Part print with two shaded views. Sizes in mm from the minimum x, y, z corner. A direction names the side the tool comes from. Give positions to 0.01 mm unless a question says otherwise; leave off trailing zeros. Loops run counter-clockwise (first coordinate to the right, second up) from the corner with the lowest first, then second, coordinate; pieces in that order, holes last. Notation, with made-up numbers: M 39,27.25 L 64,27.25 A27 ccw 64,54.25 Z; hole C -7,56 d9. An arc over 180 degrees is marked long. Answer as a JSON object with one key per item and string values. Group by question number.
1. Slice it at D-D (z = 4.4). List the corners of the cut face in (x, y), then the cut area to 3 significant figures.
2. 3-axis set-ups, long thin cutter, end or side, ignore diameter. For the marked faces 1, 2 and 3: which of +Z, -Z, +X, -X, +Y, -Y reach the whole face in a straight line?
3. Slice it at A-A (z = 2.5). List the corners of the cut face in (x, y), then the cut area to 3 significant figures.
4. Drop flat-ended pins along their axis: pin 1 Ø1 at (x, z) = (34, 4) entering from +Y; pin 2 Ø1.5 at (x, z) = (4, 3.5) entering from +Y; pin 3 Ø1.6 at (x, z) = (3, 2.5) entering from +Y; pin 4 Ø1 at (x, z) = (25, 2.5) entering from -Y. Give the stop position or say it passes through.
5. Slice it at B-B (y = 7.5). List the corners of the cut face in (x, z), then the cut area to 3 significant figures.
6. Mould opens along Y. For the marked faces 4, 5, 6 and 7 say: released by +Y, released by -Y, zero draft, split by the parting line, or undercut.
7. Slice it at C-C (x = 3). List the corners of the cut face in (y, z).
8. Drill centre lines: line 1 along X through (y, z) = (7.5, 2.05); line 2 along Z through (x, y) = (3, 8.9); line 3 along X through (y, z) = (9.6, 2.5). Where is each one in solid material? Low to high. Write a range as [from, to].
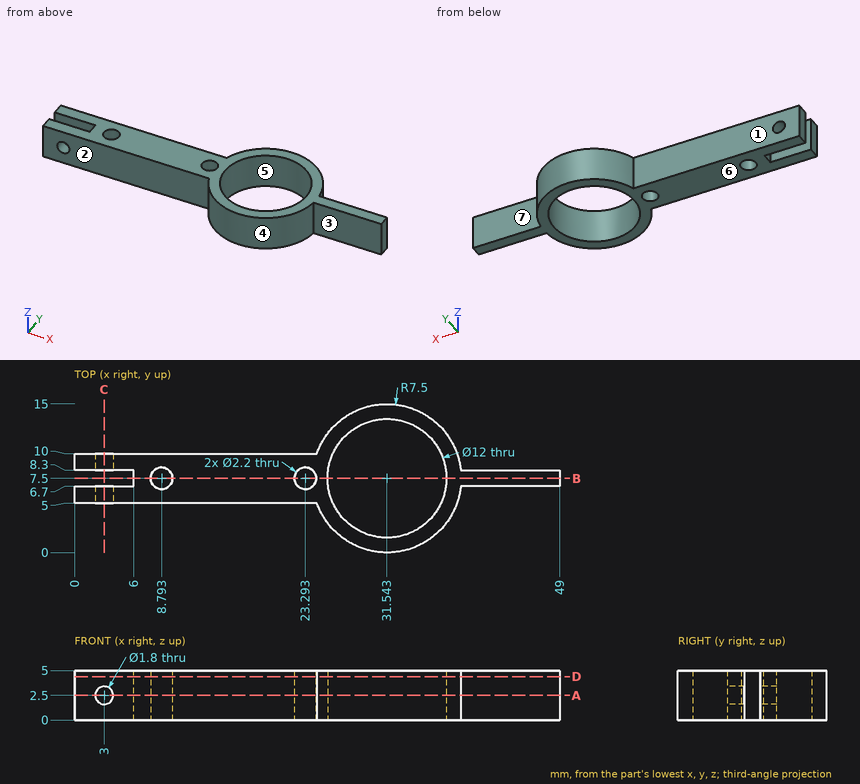
Established:
{
 "1": {"outline": "M 0,5 L 24.47,5 A7.5 ccw 39,6.7 L 49,6.7 L 49,8.3 L 39,8.3 A7.5 ccw 24.47,10 L 0,10 L 0,8.3 L 6,8.3 L 6,6.7 L 0,6.7 Z; hole C 8.79,7.5 d2.2; hole C 23.29,7.5 d2.2; hole C 31.54,7.5 d12", "area": "183 mm^2"},
 "2": {"face 1": "+Z, -Z, -X, +Y", "face 2": "+Z, -Z, -X, -Y", "face 3": "+Z, -Z, +X, -Y"},
 "3": {"outline": "M 0,5 L 2.1,5 L 2.1,6.7 L 0,6.7 Z; M 0,8.3 L 2.1,8.3 L 2.1,10 L 0,10 Z; M 3.9,5 L 24.47,5 A7.5 ccw 39,6.7 L 49,6.7 L 49,8.3 L 39,8.3 A7.5 ccw 24.47,10 L 3.9,10 L 3.9,8.3 L 6,8.3 L 6,6.7 L 3.9,6.7 Z; hole C 8.79,7.5 d2.2; hole C 23.29,7.5 d2.2; hole C 31.54,7.5 d12", "area": "177 mm^2"},
 "4": {"pin 1": "stops at y = 14.74", "pin 2": "stops at y = 10", "pin 3": "passes through", "pin 4": "stops at y = 3.06"},
 "5": {"outline": "M 6,0 L 7.69,0 L 7.69,5 L 6,5 Z; M 9.89,0 L 22.19,0 L 22.19,5 L 9.89,5 Z; M 24.39,0 L 25.54,0 L 25.54,5 L 24.39,5 Z; M 37.54,0 L 49,0 L 49,5 L 37.54,5 Z", "area": "133 mm^2"},
 "6": {"face 4": "released by -Y", "face 5": "undercut", "face 6": "zero draft", "face 7": "released by +Y"},
 "7": {"outline": "M 5,0 L 6.7,0 L 6.7,1.6 L 5,1.6 Z; M 5,3.4 L 6.7,3.4 L 6.7,5 L 5,5 Z; M 8.3,0 L 10,0 L 10,1.6 L 8.3,1.6 Z; M 8.3,3.4 L 10,3.4 L 10,5 L 8.3,5 Z"},
 "8": {"line 1": "x = [6, 7.69], [9.89, 22.19], [24.39, 25.54], [37.54, 49]", "line 2": "z = [0, 1.6], [3.4, 5]", "line 3": "x = [0, 2.1], [3.9, 25.92], [37.16, 38.74]"}
}
